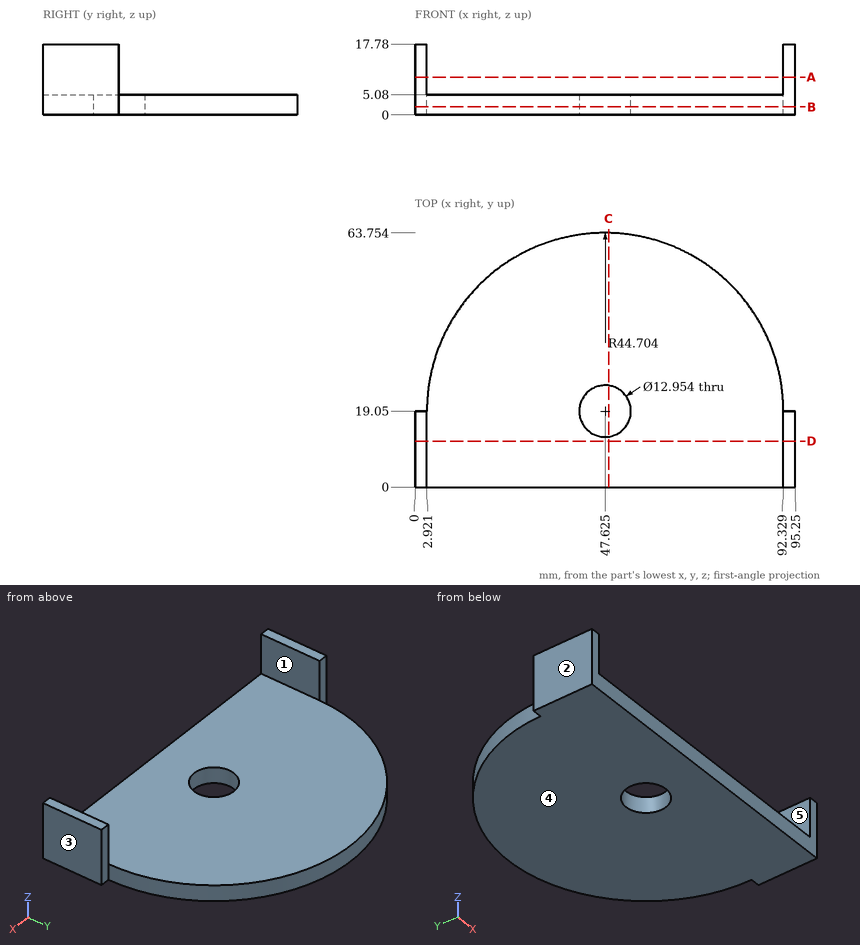
The figure shows three views and two pictorial views of one solid part (mm, origin at its lowest corner). Answer the questions. A direction names the side the tool comes from. Round coordinates to 2 decimals unless told otherwise and drop trailing zeros. Write each loop counter-clockwise with the first axis right and the second up, starting at its lowest first coordinate (ties: lowest second). Pieces come first, ordered by that corner, then holes. Notation, with made-up numbers: (-22, 16.5) - (1, 16.5) arc R18 ccw to (1, 51.5) - close; hole circle Ø2 at (7, 39). An arc over 180 degrees is marked (long way). Answer in a Markdown table with one row per item. Add a question column.
1. For the marked faces 1 and 2, determine the directions among +Z, -Z, +X, -X, +Y, -Y from which every point of the face is accessible in a straight line to the end or side of a thin tool.
2. A cutting plane is placed at C-C, the plane x = 48.5. Determine the outline of the cut face in (y, z).
3. Given pin 1 (0.9 mm diameter, centred on x = 94, z = 11.5, fed in from +Y); pin 2 (8 mm diameter, centred on x = 36, y = 45.5, fed in from +Z); pin 3 (5 mm diameter, centred on x = 39.5, z = 5, fed in from +Y), each flat-ended and moving along its own axis, determine where each tip first touches the part or whether it passes through.
4. Find the intervals of material crossed by line 1 along X through (y, z) = (5, 12.25); line 2 along Y through (x, z) = (48, 1.25); line 3 along Z through (x, y) = (74.5, 52), in increasing order. Write a range as from..to.
5. A cutting plane is placed at A-A, the plane z = 9.5. Determine the outline of the cut face in (x, y).
6. A cutting plane is placed at D-D, the plane y = 11.5. Determine the outline of the cut face in (x, z), and give its area (3 significant figures).
7. A cutting plane is placed at B-B, the plane z = 2. Determine the outline of the cut face in (x, y) (3 decimals).
8. The mould has two halves that part along X. Classify the marked faces 3, 4 and 5: +X half, -X half, draft (parallel to the pull), parting line (faces both ways), or undercut.
Worked out:
| question | item | result |
|---|---|---|
| 1 | face 1 | +Z, +Y, -Y |
| 1 | face 2 | +Z, -Z, -X, +Y, -Y |
| 2 | outline | (0, 0) - (12.63, 0) - (12.63, 5.08) - (0, 5.08) - close; (25.47, 0) - (63.75, 0) - (63.75, 5.08) - (25.47, 5.08) - close |
| 3 | pin 1 | y = 19.05 |
| 3 | pin 2 | z = 5.08 |
| 3 | pin 3 | y = 63.4 |
| 4 | line 1 | 0..2.92, 92.33..95.25 |
| 4 | line 2 | 0..12.58, 25.52..63.75 |
| 4 | line 3 | 0..5.08 |
| 5 | outline | (0, 0) - (2.92, 0) - (2.92, 19.05) - (0, 19.05) - close; (92.33, 0) - (95.25, 0) - (95.25, 19.05) - (92.33, 19.05) - close |
| 6 | outline | (0, 0) - (95.25, 0) - (95.25, 17.78) - (92.33, 17.78) - (92.33, 5.08) - (2.92, 5.08) - (2.92, 17.78) - (0, 17.78) - close |
| 6 | area | 558 mm^2 |
| 7 | outline | (0, 0) - (95.25, 0) - (95.25, 19.05) - (92.329, 19.05) arc R44.704 ccw to (2.921, 19.05) - (0, 19.05) - close; hole circle Ø12.954 at (47.625, 19.05) |
| 8 | face 3 | +X half |
| 8 | face 4 | draft |
| 8 | face 5 | undercut |
